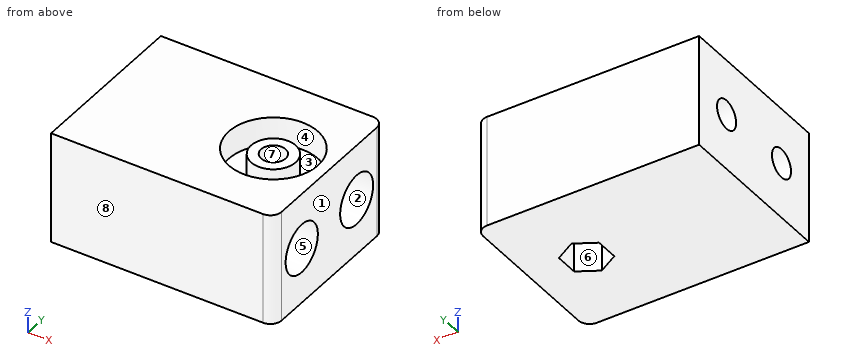
Autodesk Fusion 360 part; units mm, degrees
sketch "Sketch1" plane through (0, 0, 0) normal (0, 0, 1) x (1, 0, 0)
  line L0 (0, 0) -> (40, 0)
  line L1 (40, 0) -> (40, -30)
  line L2 (40, -30) -> (0, -30)
  line L3 (0, -30) -> (0, 0)
  line L4 (30, 0) -> (30, -30) construction
  line L5 (40, -15) -> (0, -15) construction
  circle A0 centre (30, -15) radius 8
  circle A1 centre (30, -15) radius 4
  circle A2 centre (30, -15) radius 2.2
  line L6 (33.6, -12.9215) -> (30, -10.8431)
  line L7 (30, -10.8431) -> (26.4, -12.9215)
  line L8 (26.4, -12.9215) -> (26.4, -17.0785)
  line L9 (26.4, -17.0785) -> (30, -19.1569)
  line L10 (30, -19.1569) -> (33.6, -17.0785)
  line L11 (33.6, -17.0785) -> (33.6, -12.9215)
  point P0 (30, -15)
  dimension "d1" = 40
  dimension "d2" = 30
  dimension "d3" = 10
  dimension "d4" = 15
  dimension "d5" = 16
  dimension "d6" = 8
  dimension "d7" = 4.4
  dimension "d17" = 3.6
extrude "Extrude1" add sketch "Sketch1" along normal blind 20 contours L0 L1 L2 L3
extrude "Extrude3" add sketch "Sketch1" along normal blind 15 contours A0 | A1 L6 L11 | A1 L10 L11 | A1 L6 L7 | A1 L9 L10 | A1 L7 L8 | A1 L8 L9
extrude "Extrude4" add sketch "Sketch1" along normal blind 19 contours A1 L11 | A1 L6 L7 L8 L9 L10 L11 | A1 L6 | A1 L10 | A1 L7 | A1 L9 | A1 L8 | A2
extrude "Extrude5" cut sketch "Sketch1" along normal blind 6 contours A1 L6 L7 L8 L9 L10 L11 | A1 L6 L11 | A1 L10 L11 | A1 L6 L7 | A1 L9 L10 | A1 L7 L8 | A1 L8 L9 | A2
extrude "Extrude8" cut sketch "Sketch1" along normal up to surface (13.2 mm away) from surface at 5.8 contours A2
sketch "Sketch2" plane through (40, 0, 0) normal (1, 0, 0) x (0, 1, 0)
  line L0 (-30, 0) -> (0, 0)
  line L1 (0, 0) -> (0, 20)
  line L2 (0, 20) -> (-30, 20)
  line L3 (-30, 20) -> (-30, 0)
  line L4 (-22.5, 20) -> (-22.5, 0) construction
  line L5 (-7.5, 20) -> (-7.5, 0) construction
  line L6 (-30, 10) -> (0, 10) construction
  line L7 (0, 0) -> (-30, 0) construction
  line L8 (-15, 20) -> (-15, 0) construction
  circle A0 centre (-7.5, 10) radius 2.6
  circle A1 centre (-7.5, 10) radius 4.5
  circle A2 centre (-22.5, 10) radius 2.6
  circle A3 centre (-22.5, 10) radius 4.4
  dimension "d21" = 10
  dimension "d22" = 15
  dimension "d23" = 15
  dimension "d24" = 7.5
  dimension "d25" = 5.2
  dimension "d26" = 9
  dimension "d27" = 5.2
  dimension "d28" = 8.8
extrude "Extrude6" cut sketch "Sketch2" against normal up to surface (36 mm away) contours A0 | A1 | A2 | A3
extrude "Extrude7" cut sketch "Sketch2" against normal up to surface (4 mm away) from surface at -36 contours A0 | A2
fillet "Fillet1" radius 2 2 edges at (40, 0, 10) (40, -30, 10)
Source: CAD feature listing. Evaluate the final solid. Frame: model axes, mm. Face numbers are marked on the shaded views. A direction names the side the tool comes from. Round coordinates to 2 decimals unless told otherwise and drop trailing zeros. Loops run counter-clockwise (first coordinate to the right, second up) from the corner with the lowest first, then second, coordinate; pieces in that order, holes last. Notation, with made-up numbers: M -0.5,45.5 L 41.5,45.5 A31 cw 41.5,75.5 Z; hole C 83,1.5 d9. An arc over 180 degrees is marked long. Use a Markdown table: item, result. Add a question column.
1. Contact query for flat-ended pins moving along their axis: P1, Ø2.5, axis at x = 30, y = -15, coming from the +Z side; P2, Ø7, axis at y = -22.5, z = 10, coming from the +X side; P3, Ø3.5, axis at x = 29, y = -15, coming from the -Z side; P4, Ø1, axis at x = 29, y = -13, coming from the +Z side. Output: stop coordinate, or through.
2. Reachability of the marked faces 4, 5, 6, 7 and 8 from +Z, -Z, +X, -X, +Y, -Y: full face, straight path, thin tool, end or side. Return the list, or none.
3. Section query A-A on z = 10. Return the cut outline in (x, y), then the cut area to 3 significant figures.
4. Section query C-C on y = -15. Return the cut outline in (x, z), then the cut area to 3 significant figures.
5. Section query B-B on z = 17.5. Return the cut outline in (x, y).
6. Section query D-D on x = 17. Return the cut outline in (y, z).
7. Mould query, pull axis Z, two halves, no side actions, for the marked faces 1, 2 and 3. Classes: pulls with the +Z half, pulls with the -Z half, needs draft (parallel to the pull), parting line crosses it, or undercut.
8. Line query: line 1 (Y direction, x = 21.5, z = 10.25); line 2 (Y direction, x = 30, z = 17.9); line 3 (Y direction, x = 27.5, z = 8.5). Output: solid intervals per line, ascending.
Reported:
| question | item | result |
|---|---|---|
| 1 | P1 | passes through |
| 1 | P2 | stops at x = 4 |
| 1 | P3 | stops at z = 6 |
| 1 | P4 | stops at z = 19 |
| 2 | face 4 | +Z |
| 2 | face 5 | +X |
| 2 | face 6 | -Z |
| 2 | face 7 | +Z, -Z |
| 2 | face 8 | +Z, -Z, +X, -X, -Y |
| 3 | outline | M 0,-30 L 38,-30 A2 ccw 40,-28 L 40,-26.9 L 4,-26.9 L 4,-25.1 L 0,-25.1 Z; M 0,-19.9 L 4,-19.9 L 4,-18.1 L 40,-18.1 L 40,-12 L 4,-12 L 4,-10.1 L 0,-10.1 Z; M 0,-4.9 L 4,-4.9 L 4,-3 L 40,-3 L 40,-2 A2 ccw 38,0 L 0,0 Z; hole C 30,-15 d4.4 |
| 3 | area | 501 mm² |
| 4 | outline | M 0,0 L 26.4,0 L 26.4,6 L 27.8,6 L 27.8,19 L 26,19 L 26,15 L 22,15 L 22,20 L 0,20 Z; M 32.2,6 L 33.6,6 L 33.6,0 L 40,0 L 40,20 L 38,20 L 38,15 L 34,15 L 34,19 L 32.2,19 Z |
| 4 | area | 652 mm² |
| 5 | outline | M 0,-30 L 38,-30 A2 ccw 40,-28 L 40,-2 A2 ccw 38,0 L 0,0 Z; C 30,-15 d8; hole C 30,-15 d16; hole C 30,-15 d4.4 |
| 6 | outline | M -30,0 L 0,0 L 0,20 L -30,20 Z; hole C -22.5,10 d8.8; hole C -7.5,10 d9 |
| 7 | face 1 | needs draft |
| 7 | face 2 | undercut |
| 7 | face 3 | pulls with the +Z half |
| 8 | line 1 | y = -30 to -26.89, -18.11 to -11.99, -3.01 to 0 |
| 8 | line 2 | y = -30 to -23, -19 to -17.2, -12.8 to -11, -7 to 0 |
| 8 | line 3 | y = -30 to -26.64, -18.36 to -11.74, -3.26 to 0 |
